from build123d import *

# Parameters (mm, degrees)
SKETCH_2_W               = 1.2
SKETCH_2_H               = 1.2
CUT_EXTRUDE_1_DEPTH      = 3
CUT_EXTRUDE_1_DEPTH_BACK = 3
CHAMFER_1_SIZE           = 0.4
FILLET_1_R               = 1
FILLET_2_R               = 0.4


with BuildPart() as part:
    # Эскиз1 → Повернуть1 (revolve)
    with BuildSketch(Plane(origin=(0, 0, 0), x_dir=(1, 0, 0), z_dir=(0, 1, 0))):
        Polygon((0, 0), (-2, 0), (-2, 1.8), (-1, 1.8), (-1, 8), (0, 8), align=None)
    revolve(axis=Axis((0, 0, -8), (0, 0, 1)))

    # Эскиз2 → Вырез-Вытянуть1 (cut, two sides)
    with BuildSketch(Plane(origin=(0, 0, 0), x_dir=(0, 0, -1), z_dir=(1, 0, 0))) as cut_extrude_1_sk:
        with Locations((0.6, 0)):
            Rectangle(SKETCH_2_W, SKETCH_2_H)
    extrude(amount=CUT_EXTRUDE_1_DEPTH, mode=Mode.SUBTRACT)
    extrude(cut_extrude_1_sk.sketch, amount=-CUT_EXTRUDE_1_DEPTH_BACK, mode=Mode.SUBTRACT)

    # Фаска1
    chamfer_1_edges = [part.edges().sort_by_distance(p)[0] for p in [
        (1, 0, -8),
    ]]
    chamfer(chamfer_1_edges, length=CHAMFER_1_SIZE)

    # Скругление1
    fillet_1_edges = [part.edges().sort_by_distance(p)[0] for p in [
        (0, 2, 0),
        (0, -2, 0),
    ]]
    fillet(fillet_1_edges, radius=FILLET_1_R)

    # Скругление2
    fillet_2_edges = [part.edges().sort_by_distance(p)[0] for p in [
        (1, 0, -1.8),
    ]]
    fillet(fillet_2_edges, radius=FILLET_2_R)


solid = part.part
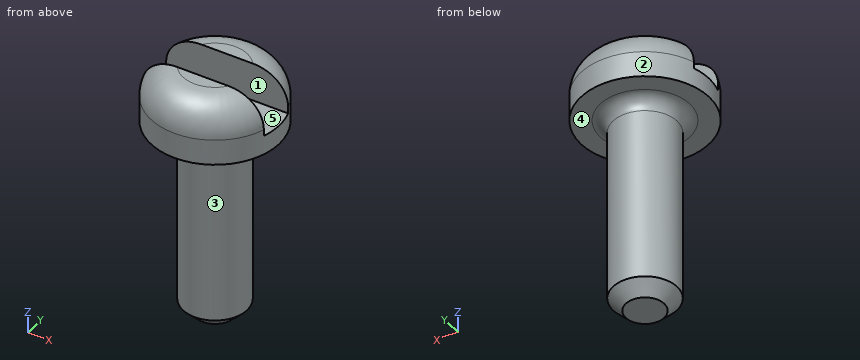
Design review of the part built by this model. Coordinates are the model's own, in mm. Face numbers are marked on the shaded views. A direction names the side the tool comes from. Coordinates: 2 decimals unless noted, no trailing zeros. Use a Markdown table: item, result.
(1) Wall thickness on probe 1 along X at (y, z) = (0.8, -7.5); probe 2 along Y at (x, z) = (-0.6, -0.75); probe 3 along Y at (x, z) = (-1, -0.5): over which ranges is each line inside the solid? List them lowest first.
Worked answers:
| item | result |
|---|---|
| probe 1 | x = -0.6 to 0.6 |
| probe 2 | y = -1.87 to -0.6, 0.6 to 1.87 |
| probe 3 | y = -1.58 to -0.6, 0.6 to 1.58 |
(2) For the marked faces 1 and 2, list the 3-axis set-ups (+Z, -Z, +X, -X, +Y, -Y) from which the entire face can be reached by the end or side of a thin tool; tool diameter is ignored.
Worked answers:
| item | result |
|---|---|
| face 1 | +Z, +X, -X |
| face 2 | +Z, -Z |
(3) For P1, Ø0.6, axis at x = 0.5, z = -0.5, coming from the -Y side; P2, Ø1, axis at x = -0.5, z = -0.5, coming from the +Y side; P3, Ø1.5, axis at y = 0, z = -4.5, coming from the -X side, all flat-tipped, find the tip position at first contact; note any pin that passes through.
Worked answers:
| item | result |
|---|---|
| P1 | stops at y = -1.94 |
| P2 | stops at y = 1.99 |
| P3 | stops at x = -1 |
(4) Draft analysis for pull direction Y (two halves, no side actions). For the marked faces 3, 4 and 5, state which applies: released by +Y, released by -Y, zero draft, split by the parting line, or undercut.
Worked answers:
| item | result |
|---|---|
| face 3 | split by the parting line |
| face 4 | zero draft |
| face 5 | undercut |
